Geometry check sheet. Reference: the model listing, model coordinates, mm. A direction names the side the tool comes from. Round coordinates to 2 decimals unless told otherwise and drop trailing zeros. Write each loop counter-clockwise with the first axis right and the second up, starting at its lowest first coordinate (ties: lowest second). Pieces come first, ordered by that corner, then holes. Notation, with made-up numbers: (-23, 61.25) -> (23, 61.25) arc R21 ccw to (23, 68.25) -> close; hole circle Ø7 at (29.25, 31). An arc over 180 degrees is marked (long way). Put each result on its own line as item: value. Start each with the question number.
Autodesk Inventor part; units mm, degrees
ref_plane "YZ Plane" through (0, 0, 0) normal (1, 0, 0) x (0, 1, 0)
ref_plane "XZ Plane" through (0, 0, 0) normal (0, 1, 0) x (-1, 0, 0)
ref_plane "XY Plane" through (0, 0, 0) normal (0, 0, 1) x (1, 0, 0)
sketch "Sketch1" plane through (0, 0, 0) normal (0, 0, 1) x (1, 0, 0)
  circle A0 centre (0, 0) radius 7.25
  circle A1 centre (0, 0) radius 12.7
  circle A2 centre (0, 0) radius 9.525 construction
  circle A3 centre (9.525, 0) radius 1.75
  circle A4 centre (-4.7625, 8.2489) radius 1.75
  circle A5 centre (-4.7625, -8.2489) radius 1.75
  dimension "d2" = 19.05
  dimension "d0" = 14.5
  dimension "d1" = 25.4
  dimension "d3" = 3.5
  dimension "d6" = 360
extrude "Extrusion1" add sketch "Sketch1" along normal blind 4.5
sketch "Sketch2" plane through (0, 0, 4.5) normal (0, 0, 1) x (1, 0, 0)
  circle A0 centre (0, 0) radius 12.7
  circle A1 centre (-4.7625, 8.2489) radius 1.75
  circle A2 centre (9.525, 0) radius 1.75
  circle A3 centre (-4.7625, -8.2489) radius 1.75
extrude "Extrusion2" add sketch "Sketch2" along normal blind 1
sketch "Sketch3" plane through (0, 0, 5.5) normal (0, 0, 1) x (1, 0, 0)
  line L0 (-4, 0.5) -> (4, 0.5)
  line L1 (4, 0.5) -> (4, -0.5)
  line L2 (4, -0.5) -> (-4, -0.5)
  line L3 (-4, -0.5) -> (-4, 0.5)
  point P0 (0, 0)
  point P1 (4, 0)
  point P2 (0, 0.5)
  dimension "d12" = 1
  dimension "d13" = 8
extrude "Extrusion3" add sketch "Sketch3" along normal blind 1.5
sketch "Sketch4" plane through (0, 0, 5.5) normal (0, 0, 1) x (1, 0, 0)
  circle A0 centre (0, 0) radius 3.5
  circle A1 centre (0, 0) radius 6
  dimension "d16" = 7
  dimension "d17" = 12
extrude "Extrusion4" add sketch "Sketch4" along normal blind 12
properties part number "AA038" material "ABS Plastic"
(1) Sectioned sample at B-B (x = 0). Record the cut outline in (y, z).
(2) Set-up check for faces 4 (the flat face through (0, 0.5, 6)), 5 (the cylindrical face through (3.35, 6.43, 2.22)), 6 (the flat face through (5.5, -5.5, 0)): record each of +Z, -Z, +X, -X, +Y, -Y from which the full face is reachable in a straight line by a thin tool's end or side.
(3) Mould release check, pull along X, two halves, no side actions. Record for faces 1 (the flat face through (0, -0.5, 6)), 2 (the flat face through (-3, -5.5, 5.5)), 3 (the cylindrical face through (-2.75, 12.4, 2.71)): +X half, -X half, draft (parallel to the pull), parting line (faces both ways), or undercut.
(4) Go/stop test with flat-tipped pins: pin 1 Ø11.5 at (x, y) = (0, 0) entering from -Z; pin 2 Ø1.2 at (x, z) = (-1, 6) entering from +Y; pin 3 Ø3 at (x, z) = (-7, 2.5) entering from -Y; pin 4 Ø3 at (x, y) = (9.525, 0) entering from -Z. Record where each tip stops, or that it passes through.
(5) Sectioned sample at A-A (y = 0). Record the cut outline in (x, z) (3 decimals).
(6) Material ranges on L1, parallel to Y at x = 0, z = 2.1; L2, parallel to X at y = 2, z = 7.5; L3, parallel to Z at x = -5.5, y = -6, recorded low to high. Write a range as from..to.
(7) Sectioned sample at D-D (x = -4.5). Record the cut outline in (y, z).
(8) Sectioned sample at C-C (z = 12.5). Record the cut outline in (x, y), and give its area (3 significant figures).
Found:
1. outline: (-12.7, 0) -> (-7.25, 0) -> (-7.25, 4.5) -> (7.25, 4.5) -> (7.25, 0) -> (12.7, 0) -> (12.7, 5.5) -> (6, 5.5) -> (6, 17.5) -> (3.5, 17.5) -> (3.5, 5.5) -> (0.5, 5.5) -> (0.5, 7) -> (-0.5, 7) -> (-0.5, 5.5) -> (-3.5, 5.5) -> (-3.5, 17.5) -> (-6, 17.5) -> (-6, 5.5) -> (-12.7, 5.5) -> close
2. face 4: +Z
2. face 5: -Z
2. face 6: -Z, +X, -X, +Y, -Y
3. face 1: undercut
3. face 2: draft
3. face 3: parting line
4. pin 1: z = 4.5
4. pin 2: y = 12.68
4. pin 3: y = -11.45
4. pin 4: through
5. outline: (-12.7, 0) -> (-7.25, 0) -> (-7.25, 4.5) -> (7.25, 4.5) -> (7.25, 0) -> (7.775, 0) -> (7.775, 5.5) -> (6, 5.5) -> (6, 17.5) -> (3.5, 17.5) -> (3.5, 7) -> (-3.5, 7) -> (-3.5, 17.5) -> (-6, 17.5) -> (-6, 5.5) -> (-12.7, 5.5) -> close; (11.275, 0) -> (12.7, 0) -> (12.7, 5.5) -> (11.275, 5.5) -> close
6. L1: -12.7..-7.25, 7.25..12.7
6. L2: -5.66..-2.87, 2.87..5.66
6. L3: 0..5.5
7. outline: (-11.88, 0) -> (-9.98, 0) -> (-9.98, 5.5) -> (-11.88, 5.5) -> close; (-6.52, 0) -> (-5.68, 0) -> (-5.68, 4.5) -> (5.68, 4.5) -> (5.68, 0) -> (6.52, 0) -> (6.52, 5.5) -> (3.97, 5.5) -> (3.97, 17.5) -> (-3.97, 17.5) -> (-3.97, 5.5) -> (-6.52, 5.5) -> close; (9.98, 0) -> (11.88, 0) -> (11.88, 5.5) -> (9.98, 5.5) -> close
8. outline: circle Ø12 at (0, 0); hole circle Ø7 at (0, 0)
8. area: 74.6 mm2
